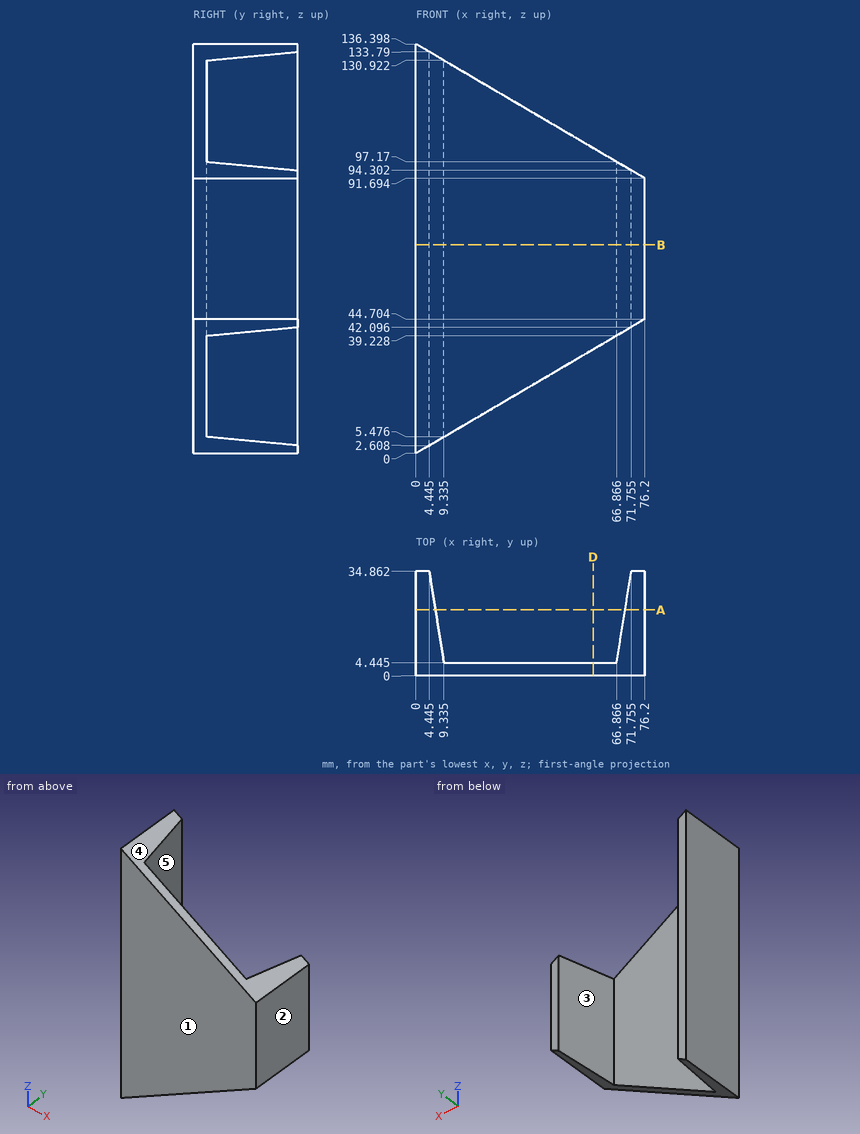
Design review of the part shown in the three views and the two pictorial views. Dimensions are in mm from the part's minimum x, y and z. A direction names the side the tool comes from. Give positions to 0.01 mm unless a question says otherwise; leave off trailing zeros. Write each loop counter-clockwise with the first axis right and the second up, starting at its lowest first coordinate (ties: lowest second). Pieces come first, ordered by that corner, then holes. Notation, with made-up numbers: (48.5, -4.5) - (89.5, -4.5) arc R23 ccw to (89.5, 32.5) - close; hole circle Ø6 at (29.5, -21). An arc over 180 degrees is marked (long way). Return JSON: item names as keys, results as strings. Group by question number.
(1) Machinability: for the marked faces 4 and 5, which of the approach directions +Z, -Z, +X, -X, +Y, -Y give a long, thin tool a straight path to every point of the face, cutting with its end or side? Answer none if there is none.
(2) Insertion check: pin 1 (3 mm diameter, centred on x = 40, z = 56.5, fed in from +Y) (1 decimal); pin 2 (3 mm diameter, centred on x = 61, z = 102.5, fed in from -Y); pin 3 (3 mm diameter, centred on y = 16, z = 31, fed in from +X); pin 4 (1.5 mm diameter, centred on x = 67.5, y = 4, fed in from -Z). Each pin has a flat end and moves straight along its axis. Give the tip position at first contact, or say it passes through.
(3) Mouldability with a two-part tool opening along X and no side actions: class the marked faces 1, 2 and 3 as +X half, -X half, draft (parallel to the pull), parting line (faces both ways), or undercut.
(4) To check wall thickness, follow probe 1 along Y at (x, z) = (63, 50) (1 decimal); probe 2 along X at (y, z) = (9, 57); probe 3 along X at (y, z) = (31.5, 57) (1 decimal). State the ranges of each line that lie inside material, in increasing order.
(5) We need section B-B, the plane z = 69.5. Give the boundary of the cut face in (x, y) (1 decimal).
(6) We need section A-A, the plane y = 22. Give the boundary of the cut face in (x, z) (1 decimal).
(7) We need section D-D, the plane x = 59. Give the boundary of the cut face in (y, z) (1 decimal).
Reported:
{
 "1": {"face 4": "+Z, +X, +Y, -Y", "face 5": "+Z, -Z, +Y"},
 "2": {"pin 1": "stops at y = 4.4", "pin 2": "passes through", "pin 3": "stops at x = 7.72", "pin 4": "stops at z = 39.16"},
 "3": {"face 1": "draft", "face 2": "+X half", "face 3": "undercut"},
 "4": {"probe 1": "y = 0 to 4.4", "probe 2": "x = 0 to 8.6, 67.6 to 76.2", "probe 3": "x = 0 to 5, 71.2 to 76.2"},
 "5": {"outline": "(0, 0) - (76.2, 0) - (76.2, 34.9) - (71.8, 34.9) - (66.9, 4.4) - (9.3, 4.4) - (4.4, 34.9) - (0, 34.9) - close"},
 "6": {"outline": "(0, 0) - (6.5, 3.8) - (6.5, 132.6) - (0, 136.4) - close; (69.7, 40.9) - (76.2, 44.7) - (76.2, 91.7) - (69.7, 95.5) - close"},
 "7": {"outline": "(0, 34.6) - (4.4, 34.6) - (4.4, 101.8) - (0, 101.8) - close"}
}
